from build123d import *

# Parameters (mm, degrees)
BOSS_EXTRUDE1_DEPTH = 45
BOSS_EXTRUDE2_START = 30
SKETCH1_3_R         = 4.5
SKETCH1_3_R_2       = 1.65
BOSS_EXTRUDE2_DEPTH = 15
SKETCH1_4_R         = 4.5
SKETCH1_4_R_2       = 1.65
BOSS_EXTRUDE3_DEPTH = 15
SKETCH5_R           = 5.5
CUT_EXTRUDE1_DEPTH  = 15
SKETCH6_R           = 2.6
CUT_EXTRUDE2_DEPTH  = 15
FILLET1_R           = 0.5
CUT_EXTRUDE3_START  = -2.5
SKETCH7_R           = 5.5
CUT_EXTRUDE3_DEPTH  = 13
SKETCH1_5_R         = 1.65
CUT_EXTRUDE4_DEPTH  = 10
SKETCH9_R           = 3.15
CUT_EXTRUDE5_DEPTH  = 10
SKETCH8_R           = 3.001117943
SKETCH8_R_2         = 3.734433125
BOSS_EXTRUDE5_DEPTH = 0.4
CUT_EXTRUDE6_START  = -2.5
SKETCH10_W          = 5.2
SKETCH10_H          = 45
CUT_EXTRUDE6_DEPTH  = 10
FILLET2_R           = 5


with BuildPart() as part:
    # Sketch1 → Boss-Extrude1 (new body)
    with BuildSketch(Plane(origin=(0, 0, 0), x_dir=(1, 0, 0), z_dir=(0, 1, 0))):
        with BuildLine():
            Line((-26.5, 4.5), (-26.5, -2))
            Line((-26.5, -2), (-4.031128874, -2))
            ThreePointArc((-4.031128874, -2), (-3.824264635, 2.371708245), (0, 4.5))
            Line((0, 4.5), (-26.5, 4.5))
        make_face()
    extrude(amount=BOSS_EXTRUDE1_DEPTH)

    # Sketch1<3> → Boss-Extrude2 (add)
    with BuildSketch(Plane(origin=(0, 0, 0), x_dir=(1, 0, 0), z_dir=(0, 1, 0)).offset(BOSS_EXTRUDE2_START)):
        Circle(SKETCH1_3_R)
        with Locations(Location((0, 0, 0), (0, 0, 270))):
            Circle(SKETCH1_3_R_2, mode=Mode.SUBTRACT)
    extrude(amount=BOSS_EXTRUDE2_DEPTH)

    # Sketch1<4> → Boss-Extrude3 (add)
    # profile 1 of 2: a face of its own
    with BuildSketch(Plane(origin=(0, 0, 0), x_dir=(1, 0, 0), z_dir=(0, 1, 0))):
        Circle(SKETCH1_4_R)
        Polygon((-2.857883832, -1.65), (0, -3.3), (2.857883832, -1.65), (2.857883832, 1.65), (0, 3.3), (-2.857883832, 1.65), align=None, mode=Mode.SUBTRACT)
    # profile 2 of 2: a face of its own
    with BuildSketch(Plane(origin=(0, 0, 0), x_dir=(1, 0, 0), z_dir=(0, 1, 0))):
        Polygon((-2.857883832, 1.65), (-2.857883832, -1.65), (0, -3.3), (2.857883832, -1.65), (2.857883832, 1.65), (0, 3.3), align=None)
        with Locations(Location((0, 0, 0), (0, 0, 270))):
            Circle(SKETCH1_4_R_2, mode=Mode.SUBTRACT)
    extrude(amount=BOSS_EXTRUDE3_DEPTH)

    # Sketch5 → Cut-Extrude1 (cut)
    with BuildSketch(Plane(origin=(0, 15, 0), x_dir=(1, 0, 0), z_dir=(0, 1, 0))):
        Circle(SKETCH5_R)
    extrude(amount=CUT_EXTRUDE1_DEPTH, mode=Mode.SUBTRACT)

    # Sketch6 → Cut-Extrude2 (cut)
    with BuildSketch(Plane.XY.offset(2)):
        with Locations((-16.5, 35)):
            Circle(SKETCH6_R)
        with Locations((-16.5, 10)):
            Circle(SKETCH6_R)
    extrude(amount=-CUT_EXTRUDE2_DEPTH, mode=Mode.SUBTRACT)

    # Fillet1
    fillet1_edges = [part.edges().sort_by_distance(p)[0] for p in [
        (-3.16227766, 22.5, -4.5),
    ]]
    fillet(fillet1_edges, radius=FILLET1_R)

    # Sketch7 → Cut-Extrude3 (cut)
    with BuildSketch(Plane(origin=(0, 0, -4.5), x_dir=(-1, 0, 0), z_dir=(0, 0, -1)).offset(CUT_EXTRUDE3_START)):
        with Locations((16.5, 35)):
            Circle(SKETCH7_R)
        with Locations((16.5, 10)):
            Circle(SKETCH7_R)
    extrude(amount=CUT_EXTRUDE3_DEPTH, mode=Mode.SUBTRACT)

    # Sketch1<5> → Cut-Extrude4 (cut)
    with BuildSketch(Plane(origin=(0, 0, 0), x_dir=(1, 0, 0), z_dir=(0, 1, 0))):
        Polygon((-2.857883832, 1.65), (-2.857883832, -1.65), (0, -3.3), (2.857883832, -1.65), (2.857883832, 1.65), (0, 3.3), align=None)
        with Locations(Location((0, 0, 0), (0, 0, 270))):
            Circle(SKETCH1_5_R, mode=Mode.SUBTRACT)
    extrude(amount=CUT_EXTRUDE4_DEPTH, mode=Mode.SUBTRACT)

    # Sketch9 → Cut-Extrude5 (cut)
    with BuildSketch(Plane(origin=(0, 45, 0), x_dir=(1, 0, 0), z_dir=(0, 1, 0))):
        with Locations(Location((0, 0, 0), (0, 0, 270))):
            Circle(SKETCH9_R)
    extrude(amount=-CUT_EXTRUDE5_DEPTH, mode=Mode.SUBTRACT)

    # Sketch8 → Boss-Extrude5 (add)
    with BuildSketch(Plane(origin=(0, 0, -2), x_dir=(-1, 0, 0), z_dir=(0, 0, -1))):
        with Locations((16.5, 35)):
            Circle(SKETCH8_R)
        with Locations((16.5, 10)):
            Circle(SKETCH8_R_2)
    extrude(amount=-BOSS_EXTRUDE5_DEPTH)

    # Sketch10 → Cut-Extrude6 (cut)
    with BuildSketch(Plane(origin=(0, 0, -4.5), x_dir=(-1, 0, 0), z_dir=(0, 0, -1)).offset(CUT_EXTRUDE6_START)):
        with Locations((23.9, 22.5)):
            Rectangle(SKETCH10_W, SKETCH10_H)
    extrude(amount=-CUT_EXTRUDE6_DEPTH, mode=Mode.SUBTRACT)

    # Fillet2
    fillet2_edges = [part.edges().sort_by_distance(p)[0] for p in [
        (-26.5, 45, -3.25),
        (-21.3, 45, 0),
        (-26.5, 0, -3.25),
        (-21.3, 0, 0),
    ]]
    fillet(fillet2_edges, radius=FILLET2_R)


solid = part.part
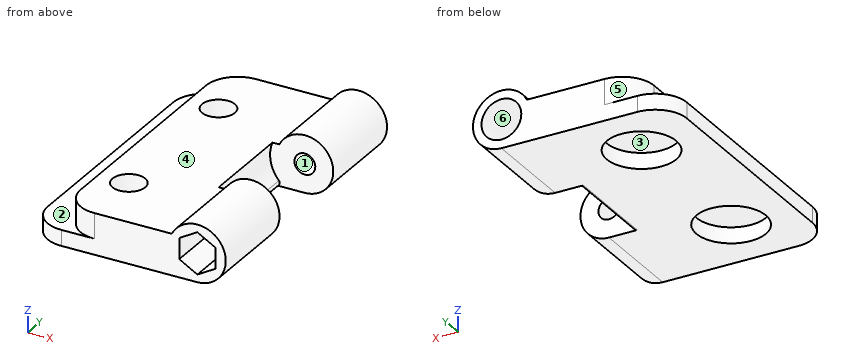
Work out the finished part from the listing and answer in its coordinate system (mm). Face numbers are marked on the shaded views. A direction names the side the tool comes from. Round coordinates to 2 decimals unless told otherwise and drop trailing zeros. Write each loop counter-clockwise with the first axis right and the second up, starting at its lowest first coordinate (ties: lowest second). Pieces come first, ordered by that corner, then holes. Notation, with made-up numbers: (60.25, -26.5) -> (88.25, -26.5) arc R13 ccw to (88.25, -21.5) -> close; hole circle Ø5 at (-6, 63). An arc over 180 degrees is marked (long way). Answer as CSV lines item,"result". Start each with the question number.
(1) Each of these flat-tipped pins is pushed along its axis until it touches: pin 1 (17.5 mm diameter, centred on x = -16.5, y = 35, fed in from +Z); pin 2 (1.5 mm diameter, centred on y = 12, z = 2.5, fed in from +X); pin 3 (1.6 mm diameter, centred on y = 5, z = 0.5, fed in from -X). Where does it stop, or does it pass through?
(2) A tool of negligible diameter and unlimited length cuts with its end or side. For the marked faces 4, 5 and 6, from which of +Z, -Z, +X, -X, +Y, -Y can it reach the whole face along a straight path? Write none if from no direction.
(3) Find the intervals of material crossed by probe 1 along Y at (x, z) = (-16.5, -0.75); probe 2 along Y at (x, z) = (-4, -1.5); probe 3 along Y at (x, z) = (-13, -2.25), in increasing order.
(4) The mould has two halves that part along Z. Classify the marked faces 1, 2 and 3: +Z half, -Z half, draft (parallel to the pull), parting line (faces both ways), or undercut.
(5) The part is cut by section B-B, the plane y = 12. Give the vertices of the cut face in (x, z), then the cut area to 3 significant figures.
(6) The part is cut by section A-A, the plane z = 0. Give the vertices of the cut face in (x, y), then the cut area to 3 significant figures.
(7) The part is cut by section D-D, the plane x = -7. Give the vertices of the cut face in (y, z), then the cut area to 4 significant figures.
(8) The part is cut by section C-C, the plane y = 38.5. Give the vertices of the cut face in (x, z).
Output values:
1,pin 1,"stops at z = 2"
1,pin 2,"stops at x = 4.15"
1,pin 3,"stops at x = -21.3"
2,face 4,"+Z, -X, +Y, -Y"
2,face 5,"+Z, -X, +Y"
2,face 6,"+Y"
3,probe 1,"y = 0 to 7.4, 12.6 to 32.4, 37.6 to 45"
3,probe 2,"y = 0 to 15, 30 to 45"
3,probe 3,"y = 0 to 5.76, 14.24 to 30.76, 39.24 to 45"
4,face 1,"undercut"
4,face 2,"+Z half"
4,face 3,"-Z half"
5,outline,"(-26.5, -4.5) -> (-21.62, -4.5) -> (-21.62, -2) -> (-26.5, -2) -> close; (-21.3, -2) -> (-11.38, -2) -> (-11.38, -4.5) -> (0, -4.5) arc R4.5 ccw (long way) to (-4.03, 2) -> (-14.84, 2) -> (-14.84, -1.6) -> (-18.16, -1.6) -> (-18.16, 2) -> (-21.3, 2) -> close; hole circle Ø3.3 at (0, 0)"
5,area,"144 mm²"
6,outline,"(-21.3, 5) arc R5 ccw to (-16.3, 0) -> (-2.86, 0) -> (-2.86, 10) -> (-1.65, 10) -> (-1.65, 15) -> (-5.5, 15) -> (-5.5, 30) -> (-1.65, 30) -> (-1.65, 35) -> (-3.15, 35) -> (-3.15, 45) -> (-16.3, 45) arc R5 ccw to (-21.3, 40) -> close; (1.65, 10) -> (2.86, 10) -> (2.86, 0) -> (4.5, 0) -> (4.5, 15) -> (1.65, 15) -> close; (1.65, 30) -> (4.5, 30) -> (4.5, 45) -> (3.15, 45) -> (3.15, 35) -> (1.65, 35) -> close; hole circle Ø5.2 at (-16.5, 10); hole circle Ø5.2 at (-16.5, 35)"
6,area,"805 mm²"
7,outline,"(0, -4.5) -> (45, -4.5) -> (45, 2) -> (0, 2) -> close"
7,area,"292.5 mm²"
8,outline,"(-26.5, -4.5) -> (-20.74, -4.5) -> (-20.74, -2) -> (-12.26, -2) -> (-12.26, -4.5) -> (0, -4.5) arc R4.5 ccw (long way) to (-4.03, 2) -> (-21.3, 2) -> (-21.3, -2) -> (-26.5, -2) -> close; hole circle Ø6.3 at (0, 0)"
